Could you check a few things on this model? Use its own coordinates, in mm. A direction names the side the tool comes from. Round coordinates to 2 decimals unless told otherwise and drop trailing zeros. Loops run counter-clockwise (first coordinate to the right, second up) from the corner with the lowest first, then second, coordinate; pieces in that order, holes last. Notation, with made-up numbers: (18.5, -39) -> (52.5, -39) arc R20 cw to (52.5, -22) -> close; hole circle Ø7 at (68.5, 1). An arc over 180 degrees is marked (long way). Put each result on its own line as item: value. Start each with the question number.
1. Which directions (+Z, -Z, +X, -X, +Y, -Y) give clear straight access to the entire face, cutting with the end or side of a thin tool? Please do faces 1 (the flat face through (-40, -56, 22.86)), 2 (the conical face through (-18.867, 84.964, -0.123)), 3 (the flat face through (-40, -56, 2.54)), 4 (the cylindrical face through (24.428, 70.543, 12.558)).
2. Imagine slicing it at A-A, the plane x = 0. Please give me the cut outline in (y, z), and give its area (3 significant figures).
3. I need wall thicknesses on line 1 (Y direction, x = 0, z = 7.75); line 2 (X direction, y = -36.5, z = 1); line 3 (Z direction, x = 58, y = 67.5). Which ranges of each line are inside material? Lowest first, please. Write a range as [from, to].
4. If we mould it in two halves opening along Y, with no side actions, what happens to faces 5 (the cylindrical face through (20.648, 92.985, -3.792)), 6 (the flat face through (43, -64, -5.08)), 7 (the cylindrical face through (36.868, 57.827, 12.558))? For each: pulls with the +Y half, pulls with the -Y half, needs draft (parallel to the pull), parting line crosses it, or undercut.
5. Imagine slicing it at C-C, the plane z = 14. Please give me the cut outline in (x, y).
6. I'm going to push flat-ended pins straight in: P1, Ø6, axis at x = -21, z = 6.5, coming from the -Y side; P2, Ø2, axis at y = 37, z = 17.5, coming from the -X side; P3, Ø12, axis at x = -37.5, z = 22.5, coming from the -Y side. Where does each tip first touch, or does it pass through?
```python
from build123d import *

# Parameters (mm, degrees)
SKETCH1_R           = 82.55
BOSS_EXTRUDE1_DEPTH = 25.4
SKETCH2_R           = 68.58
CUT_EXTRUDE1_DEPTH  = 25.4
SKETCH3_R           = 76.2
CUT_EXTRUDE2_DEPTH  = 2.54
CUT_EXTRUDE3_START  = -2.54
SKETCH4_R           = 76.2
CUT_EXTRUDE3_DEPTH  = 2.54
CHAMFER5_SIZE       = 0.254
CHAMFER6_SIZE       = 0.254
SKETCH6_R           = 2.54
CUT_EXTRUDE4_DEPTH  = 120.474537036
SKETCH7_R           = 95.25
SKETCH7_R_2         = 76.2
BOSS_EXTRUDE2_DEPTH = 25.4
SKETCH9_R           = 95.25
SKETCH9_R_2         = 76.2
BOSS_EXTRUDE3_DEPTH = 5.08


with BuildPart() as part:
    # Sketch1 → Boss-Extrude1 (new body)
    with BuildSketch(Plane.XY):
        Circle(SKETCH1_R)
    extrude(amount=BOSS_EXTRUDE1_DEPTH)

    # Sketch2 → Cut-Extrude1 (cut)
    with BuildSketch(Plane.XY):
        Circle(SKETCH2_R)
    extrude(amount=CUT_EXTRUDE1_DEPTH, mode=Mode.SUBTRACT)

    # Sketch3 → Cut-Extrude2 (cut)
    with BuildSketch(Plane.XY):
        Circle(SKETCH3_R)
    extrude(amount=CUT_EXTRUDE2_DEPTH, mode=Mode.SUBTRACT)

    # Sketch4 → Cut-Extrude3 (cut)
    with BuildSketch(Plane.XY.offset(25.4).offset(CUT_EXTRUDE3_START)):
        Circle(SKETCH4_R)
    extrude(amount=CUT_EXTRUDE3_DEPTH, mode=Mode.SUBTRACT)

    # Chamfer5
    chamfer5_edges = [part.edges().sort_by_distance(p)[0] for p in [
        (-82.55, 0, 0),
    ]]
    chamfer(chamfer5_edges, length=CHAMFER5_SIZE)

    # Chamfer6
    chamfer6_edges = [part.edges().sort_by_distance(p)[0] for p in [
        (-82.55, 0, 25.4),
    ]]
    chamfer(chamfer6_edges, length=CHAMFER6_SIZE)

    # Sketch6 → Cut-Extrude4 (cut, through all)
    with BuildSketch(Plane.XY):
        with Locations((68.024348819, 24.758838175)):
            Circle(SKETCH6_R)
        with Locations((-68.024348819, -24.758838175)):
            Circle(SKETCH6_R)
        with Locations((24.758838175, 68.024348819)):
            Circle(SKETCH6_R)
        with Locations((-24.758838175, -68.024348819)):
            Circle(SKETCH6_R)
    extrude(amount=CUT_EXTRUDE4_DEPTH, mode=Mode.SUBTRACT)

    # Sketch7 → Boss-Extrude2 (add)
    with BuildSketch(Plane(origin=(0, 0, 0), x_dir=(-1, 0, 0), z_dir=(0, 0, -1))):
        Circle(SKETCH7_R)
        with Locations(Location((0, 0, 0), (0, 0, 180))):
            Circle(SKETCH7_R_2, mode=Mode.SUBTRACT)
    extrude(amount=-BOSS_EXTRUDE2_DEPTH)

    # Sketch9 → Boss-Extrude3 (add)
    with BuildSketch(Plane.XY.offset(25.4)):
        with Locations(Location((0, 0, 0), (0, 0, 180))):
            Circle(SKETCH9_R)
        Circle(SKETCH9_R_2, mode=Mode.SUBTRACT)
    boss_extrude3 = extrude(amount=BOSS_EXTRUDE3_DEPTH)

    # Mirror1: Boss-Extrude3 across plane
    add(boss_extrude3.mirror(Plane(origin=(0, 0, 12.7), x_dir=(1, 0, 0), z_dir=(0, 0, -1))))

    # Sketch10 → Cut-Revolve1 (revolve, cut)
    with BuildSketch(Plane(origin=(0, 0, 0), x_dir=(0, 0, -1), z_dir=(1, 0, 0)), mode=Mode.PRIVATE) as cut_revolve1_sk:
        Polygon((0, 86.614), (-25.4, 86.614), (-27.94, 95.25), (2.54, 95.25), align=None)
    revolve(cut_revolve1_sk.sketch.rotate(Axis((0, 0, 22.86), (0, 0, -1)), 90), axis=Axis((0, 0, 22.86), (0, 0, -1)), mode=Mode.SUBTRACT)


solid = part.part
```
Entries:
1. face 1: +Z
1. face 2: none
1. face 3: -Z
1. face 4: +Z, -Z
2. outline: (-95.25, -5.08) -> (-76.2, -5.08) -> (-76.2, 2.54) -> (-68.58, 2.54) -> (-68.58, 22.86) -> (-76.2, 22.86) -> (-76.2, 30.48) -> (-95.25, 30.48) -> (-95.25, 27.94) -> (-86.61, 25.4) -> (-86.61, 0) -> (-95.25, -2.54) -> close; (68.58, 2.54) -> (76.2, 2.54) -> (76.2, -5.08) -> (95.25, -5.08) -> (95.25, -2.54) -> (86.61, 0) -> (86.61, 25.4) -> (95.25, 27.94) -> (95.25, 30.48) -> (76.2, 30.48) -> (76.2, 22.86) -> (68.58, 22.86) -> close
2. area: 1,180 mm^2
3. line 1: [-86.61, -68.58], [68.58, 86.61]
3. line 2: [-78.55, -66.89], [66.89, 78.55]
3. line 3: [-5.08, -0.7], [26.1, 30.48]
4. face 5: parting line crosses it
4. face 6: needs draft
4. face 7: undercut
5. outline: circle Ø173.23 at (0, 0); hole circle Ø5.08 at (-68.02, -24.76); hole circle Ø137.16 at (0, 0); hole circle Ø5.08 at (-24.76, -68.02); hole circle Ø5.08 at (24.76, 68.02); hole circle Ø5.08 at (68.02, 24.76)
6. P1: y = -84.72
6. P2: x = -78.78
6. P3: y = -88.6
